Model file for the job. Use its own axes, mm. Face numbers are marked on the shaded views. Give positions to 0.01 mm unless a question says otherwise; leave off trailing zeros. Write each loop counter-clockwise with the first axis right and the second up, starting at its lowest first coordinate (ties: lowest second). Pieces come first, ordered by that corner, then holes. Notation, with made-up numbers: (-12.75, 26) - (2.25, 26) arc R8 cw to (2.25, 37) - close; hole circle Ø1 at (16, 60.5). An arc over 180 degrees is marked (long way). One line per item, written item: value. Start each with the question number.
(1) Cut at C-C, the plane x = 37.5. List the corners of the cut face in (y, z), and give its area (3 significant figures).
(2) Drop flat-ended pins along their axis: P1, Ø1.5, axis at x = 30.5, y = 1.5, coming from the -Z side; P2, Ø7.5, axis at x = 15, y = 3.5, coming from the +Z side. Give the stop position or say it passes through.
(3) Cut at D-D, the plane x = -52.5. List the corners of the cut face in (y, z).
(4) Cut at B-B, the plane z = 6.25. List the corners of the cut face in (x, y).
(5) Mould opens along X. For the marked faces 1 and 2 say: pulls with the +X half, pulls with the -X half, needs draft (parallel to the pull), parting line crosses it, or undercut.
(6) Probe L1, parallel to X at y = 1.5, z = 4; L2, parallel to Y at x = -67.5, z = 3.85; L3, parallel to Y at x = -52.5, z = 3.6. List the from-to ranges inside material, lowest first.
(7) Cut at A-A, the plane x = -22.5. List the corners of the cut face in (y, z), and give its area (3 significant figures).
from build123d import *

# Parameters (mm, degrees)
F0_W     = 150
F0_H     = 15
F0_R     = 4.5
F0_R_2   = 4.75
F0_R_3   = 5
F0_R_4   = 5.25
F0_R_5   = 5.5
F1_DEPTH = 5
F2_R     = 7.49999
F3_R     = 3
F3_R_2   = 2.5
F3_R_3   = 2.75
F3_R_4   = 2.25
F3_R_5   = 2
F4_DEPTH = 10


# Not quite as in the source:
# - a fillet or chamfer is up to 0.001 mm smaller than in the source, because OpenCascade refuses the exact size


with BuildPart() as f1:
    # F0 (on Top) → F1 (new body)
    with BuildSketch(Plane.XY):
        Rectangle(F0_W, F0_H)
        with Locations((-67.5, 0)):
            Circle(F0_R, mode=Mode.SUBTRACT)
        with Locations((-52.5, 0)):
            Circle(F0_R_2, mode=Mode.SUBTRACT)
        with Locations((-37.5, 0)):
            Circle(F0_R_3, mode=Mode.SUBTRACT)
        with Locations((-22.5, 0)):
            Circle(F0_R_4, mode=Mode.SUBTRACT)
        with Locations((-7.5, 0)):
            Circle(F0_R_5, mode=Mode.SUBTRACT)
    extrude(amount=F1_DEPTH)

    # F2 (radius 7.5 in the source; OpenCascade refuses exactly that, so slightly less here)
    f2_edges = [f1.edges().sort_by_distance(p)[0] for p in [
        (-75, -7.5, 2.5),
        (-75, 7.5, 2.5),
        (75, -7.5, 2.5),
        (75, 7.5, 2.5),
    ]]
    fillet(f2_edges, radius=F2_R)

    # F3 (on Top) → F4 (join)
    with BuildSketch(Plane.XY):
        with Locations((67.5, 0)):
            Circle(F3_R)
        with Locations((37.5, 0)):
            Circle(F3_R_2)
        with Locations((52.5, 0)):
            Circle(F3_R_3)
        with Locations((22.5, 0)):
            Circle(F3_R_4)
        with Locations((7.5, 0)):
            Circle(F3_R_5)
    extrude(amount=F4_DEPTH)


solid = f1.part
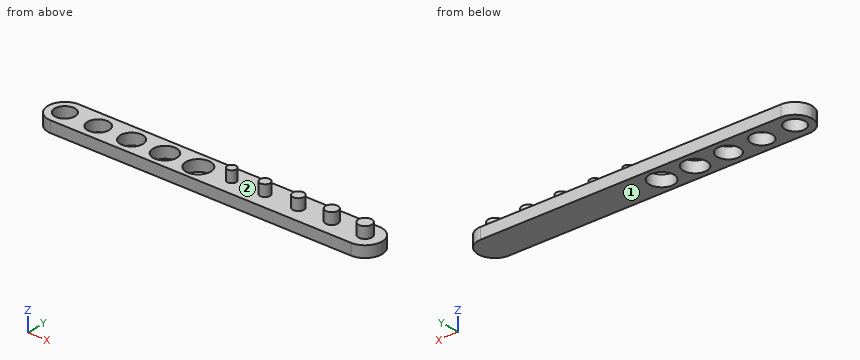
Answers follow:
1. outline: (-7.5, 0) - (7.5, 0) - (7.5, 5) - (2.5, 5) - (2.5, 10) - (-2.5, 10) - (-2.5, 5) - (-7.5, 5) - close
1. area: 100 mm²
2. P1: stops at z = 0
2. P2: stops at z = 5
3. outline: (-7.5, 0) - (-4.75, 0) - (-4.75, 5) - (-7.5, 5) - close; (4.75, 0) - (7.5, 0) - (7.5, 5) - (4.75, 5) - close
4. outline: circle Ø4 at (7.5, 0); circle Ø4.5 at (22.5, 0); circle Ø5 at (37.5, 0); circle Ø5.5 at (52.5, 0); circle Ø6 at (67.5, 0)
5. face 1: needs draft
5. face 2: undercut
6. L1: x = -74.85 to -71.74, -63.26 to -57.01, -47.99 to -42.27, -32.73 to -27.53, -17.47 to -12.79, -2.21 to 74.85
6. L2: y = -7.5 to -4.5, 4.5 to 7.5
6. L3: y = -7.5 to -4.75, 4.75 to 7.5
7. outline: (-7.5, 0) - (-5.25, 0) - (-5.25, 5) - (-7.5, 5) - close; (5.25, 0) - (7.5, 0) - (7.5, 5) - (5.25, 5) - close
7. area: 22.5 mm²
